Verification items for the finished model (mm, model axes). Face numbers are marked on the shaded views. A direction names the side the tool comes from. Round coordinates to 2 decimals unless told otherwise and drop trailing zeros. Write each loop counter-clockwise with the first axis right and the second up, starting at its lowest first coordinate (ties: lowest second). Pieces come first, ordered by that corner, then holes. Notation, with made-up numbers: (12.5, -36.75) - (57.5, -36.75) arc R29 cw to (57.5, -12.75) - close; hole circle Ø11 at (2.5, 38). An arc over 180 degrees is marked (long way). Answer as a JSON object with one key per item and string values.
```python
from build123d import *

# Parameters (mm, degrees)
F1_DEPTH = 35
F2_SIZE  = 1.5


with BuildPart() as f1:
    # F0 (on Right) → F1 (new body)
    with BuildSketch(Plane.YZ):
        Polygon((43.557955, -26.808144), (29.057955, -26.808144), (29.057955, -36.808144), (37.657955, -36.808144), (37.657955, -34.458144), (34.957955, -34.458144), (34.957955, -31.058144), (40.057955, -31.058144), (40.057955, -32.958144), (48.057955, -32.958144), (48.057955, -31.058144), (53.157955, -31.058144), (53.157955, -34.458144), (50.457955, -34.458144), (50.457955, -36.808144), (59.057955, -36.808144), (59.057955, -26.808144), (44.557955, -26.808144), align=None)
    extrude(amount=-F1_DEPTH)

    # F2
    f2_edges = [f1.edges().sort_by_distance(p)[0] for p in [
        (-17.5, 59.057955, -36.808144),
        (-17.5, 48.057955, -32.958144),
        (-17.5, 40.057955, -32.958144),
        (-17.5, 29.057955, -36.808144),
    ]]
    chamfer(f2_edges, length=F2_SIZE)


solid = f1.part
```
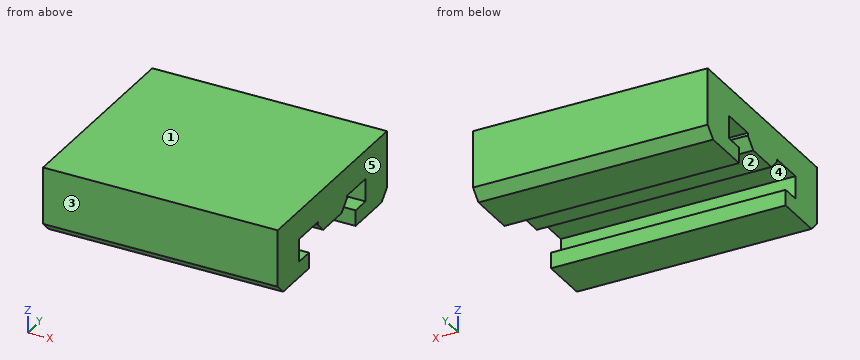
1. Cross-section at A-A (x = -20). Record the boundary of the cut face in (y, z).
Completed:
{"outline": "(29.06, -35.31) - (30.56, -36.81) - (37.66, -36.81) - (37.66, -34.46) - (34.96, -34.46) - (34.96, -31.06) - (40.06, -31.06) - (40.06, -31.46) - (41.56, -32.96) - (46.56, -32.96) - (48.06, -31.46) - (48.06, -31.06) - (53.16, -31.06) - (53.16, -34.46) - (50.46, -34.46) - (50.46, -36.81) - (57.56, -36.81) - (59.06, -35.31) - (59.06, -26.81) - (29.06, -26.81) - close"}
2. Cross-section at C-C (y = 43). Record the boundary of the cut face in (x, z), plus the area to 3 significant figures.
Completed:
{"outline": "(-35, -32.96) - (0, -32.96) - (0, -26.81) - (-35, -26.81) - close", "area": "215 mm^2"}
3. Material ranges on probe 1 along Y at (x, z) = (-9, -35); probe 2 along Z at (x, y) = (-31, 52.75); probe 3 along Y at (x, z) = (-1.5, -34), recorded low to high. Write a range as from..to.
Completed:
{"probe 1": "y = 29.06..37.66, 50.46..59.06", "probe 2": "z = -36.81..-34.46, -31.06..-26.81", "probe 3": "y = 29.06..34.96, 53.16..59.06"}
4. Access from +Z, -Z, +X, -X, +Y, -Y to the whole of each face (thin tool, end or side, straight path). Record for the marked faces 4 and 5.
Completed:
{"face 4": "+X, -X", "face 5": "+Z, -Z, +X, +Y, -Y"}
5. Mould release check, pull along Y, two halves, no side actions. Record for the marked faces 1, 2 and 3: released by +Y, released by -Y, zero draft, split by the parting line, or undercut.
Completed:
{"face 1": "zero draft", "face 2": "undercut", "face 3": "released by -Y"}
6. Cross-section at B-B (y = 49.25). Record the boundary of the cut face in (x, z).
Completed:
{"outline": "(-35, -31.06) - (0, -31.06) - (0, -26.81) - (-35, -26.81) - close"}
7. Go/stop test with flat-tipped pins: pin 1 (2.5 mm diameter, centred on x = -17, y = 43, fed in from -Z); pin 2 (1.5 mm diameter, centred on y = 36, z = -35, fed in from +X); pin 3 (1.2 mm diameter, centred on x = -24.5, z = -36, fed in from +Y). Record where each tip stops, or that it passes through.
Completed:
{"pin 1": "stops at z = -32.96", "pin 2": "stops at x = 0", "pin 3": "stops at y = 58.97"}
